Verification items for the finished model (mm, model axes). A direction names the side the tool comes from. Give positions to 0.01 mm unless a question says otherwise; leave off trailing zeros. Write each loop counter-clockwise with the first axis right and the second up, starting at its lowest first coordinate (ties: lowest second). Pieces come first, ordered by that corner, then holes. Notation, with made-up numbers: (14, -28.5) -> (50, -28.5) arc R20 cw to (50, 7.5) -> close; hole circle Ø5 at (-16, -38.5). An arc over 180 degrees is marked (long way). Answer as CSV lines item,"result". Start each with the question number.
1) Material ranges on L1, parallel to X at y = -5, z = 215; L2, parallel to Z at x = -30.5, y = -1.25; L3, parallel to X at y = -3.5, z = 236.5, recorded low to high.
2) Tool access check on faces 1 (the flat face through (32, -4, 188.594)), 2 (the flat face through (97, -4, 228.594)). Record the directions out of +Z, -Z, +X, -X, +Y, -Y that give a thin tool (end or side, any length) a straight path to the whole face; none if there is none.
3) Sectioned sample at B-B on x = -29. Record the cut outline in (y, z).
4) Sectioned sample at A-A on y = -1.75. Give the number of separate pieces and of enclosed holes in the cut face, and give its area (3 significant figures).
5) Gauge pin test, flat ends, axial feed: pin 1 Ø2.5 at (x, y) = (-33, -6) entering from +Z; pin 2 Ø4 at (y, z) = (-5.5, 235.5) entering from -X; pin 3 Ø2.5 at (y, z) = (-3.5, 233) entering from +X; pin 4 Ø2 at (x, z) = (-17.04, 213.59) entering from +Y. Record the tip position at first contact, or that the pin passes through.
6) Mould release check, pull along X, two halves, no side actions. Record for faces 3 (the flat face through (32, -8, 214)), 4 (the flat face through (92.961, -4, 234)), 5 (the cylindrical face through (-42.032, -4.056, 191.446)): released by +X, released by -X, zero draft, split by the parting line, or undercut.
```python
from build123d import *

# Parameters (mm, degrees)
F0_R     = 1.65
F1_DEPTH = 8
F2_R     = 9.99999


# Not quite as in the source:
# - a fillet or chamfer is up to 0.001 mm smaller than in the source, because OpenCascade refuses the exact size


with BuildPart() as f1:
    # F0 (on Front) → F1 (new body)
    with BuildSketch(Plane.XZ):
        Polygon((-27.0393844694, 188.5941594839), (92.9606155306, 188.5941594839), (110.9606155306, 188.5941594839), (110.9606155306, 238.5941594839), (100.9606155306, 238.5941594839), (100.9606155306, 228.5941594839), (92.9606155306, 228.5941594839), (92.9606155306, 238.5941594839), (-27.0393844694, 238.5941594839), (-27.0393844694, 228.5941594839), (-35.0393844694, 228.5941594839), (-35.0393844694, 238.5941594839), (-45.0393844694, 238.5941594839), (-45.0393844694, 188.5941594839), align=None)
        with Locations((-17.0393844694, 213.5941594839)):
            Circle(F0_R, mode=Mode.SUBTRACT)
        with Locations((82.9606155306, 213.5941594839)):
            Circle(F0_R, mode=Mode.SUBTRACT)
    extrude(amount=F1_DEPTH)

    # F2 (radius 10 in the source; OpenCascade refuses exactly that, so slightly less here)
    f2_edges = [f1.edges().sort_by_distance(p)[0] for p in [
        (-45.039384, -4, 238.594159),
        (-45.039384, -4, 188.594159),
        (110.960616, -4, 188.594159),
        (110.960616, -4, 238.594159),
    ]]
    fillet(f2_edges, radius=F2_R)


solid = f1.part
```
Ans:
1,L1,"x = -45.04 to -17.9, -16.18 to 82.1, 83.82 to 110.96"
1,L2,"z = 188.59 to 228.59"
1,L3,"x = -41.16 to -35.04, -27.04 to 92.96, 100.96 to 107.08"
2,face 1,"-Z, +X, -X, +Y, -Y"
2,face 2,"+Z, +Y, -Y"
3,outline,"(-8, 188.59) -> (0, 188.59) -> (0, 228.59) -> (-8, 228.59) -> close"
4,separate pieces,"1"
4,enclosed holes,"2"
4,area,"7,540 mm²"
5,pin 1,"stops at z = 228.59"
5,pin 2,"stops at x = -43.75"
5,pin 3,"stops at x = 110.45"
5,pin 4,"passes through"
6,face 3,"zero draft"
6,face 4,"undercut"
6,face 5,"released by -X"
